Verification items for the finished model (mm, model axes). A direction names the side the tool comes from. Round coordinates to 2 decimals unless told otherwise and drop trailing zeros. Loops run counter-clockwise (first coordinate to the right, second up) from the corner with the lowest first, then second, coordinate; pieces in that order, holes last. Notation, with made-up numbers: (10, 3) -> (56, 3) arc R14 ccw to (56, 20) -> close; hole circle Ø6 at (84.5, -39). An arc over 180 degrees is marked (long way). Use a Markdown table: item, result. Add a question column.
```python
from build123d import *

# Parameters (mm, degrees)
SKETCH1_W           = 45
SKETCH1_H           = 20
BOSS_EXTRUDE1_DEPTH = 1
SKETCH2_R           = 8.5
BOSS_EXTRUDE2_DEPTH = 10
SKETCH3_R           = 7
CUT_EXTRUDE1_DEPTH  = 1
SKETCH4_W           = 1
SKETCH4_H           = 7
BOSS_EXTRUDE3_DEPTH = 1


with BuildPart() as part:
    # Sketch1 → Boss-Extrude1 (new body)
    with BuildSketch(Plane(origin=(0, 0, 0), x_dir=(1, 0, 0), z_dir=(0, 1, 0))):
        Rectangle(SKETCH1_W, SKETCH1_H)
    extrude(amount=BOSS_EXTRUDE1_DEPTH)

    # Sketch2 → Boss-Extrude2 (add)
    with BuildSketch(Plane(origin=(0, 1, 0), x_dir=(1, 0, 0), z_dir=(0, 1, 0))):
        with Locations(Location((-13, 0, 0), (0, 0, 270))):
            Circle(SKETCH2_R)
        with Locations(Location((13, 0, 0), (0, 0, 270))):
            Circle(SKETCH2_R)
    extrude(amount=BOSS_EXTRUDE2_DEPTH)

    # Sketch3 → Cut-Extrude1 (cut)
    with BuildSketch(Plane(origin=(0, 11, 0), x_dir=(1, 0, 0), z_dir=(0, 1, 0))):
        with Locations(Location((-13, 0, 0), (0, 0, 270))):
            Circle(SKETCH3_R)
        with Locations(Location((13, 0, 0), (0, 0, 270))):
            Circle(SKETCH3_R)
    extrude(amount=-CUT_EXTRUDE1_DEPTH, mode=Mode.SUBTRACT)

    # Sketch4 → Boss-Extrude3 (add)
    with BuildSketch(Plane(origin=(0, 1, 0), x_dir=(1, 0, 0), z_dir=(0, 1, 0))):
        with Locations((-1, 11.5)):
            Rectangle(SKETCH4_W, SKETCH4_H)
        with Locations((-3, 11.5)):
            Rectangle(SKETCH4_W, SKETCH4_H)
        with Locations((3, 11.5)):
            Rectangle(SKETCH4_W, SKETCH4_H)
        with Locations((1, 11.5)):
            Rectangle(SKETCH4_W, SKETCH4_H)
    extrude(amount=BOSS_EXTRUDE3_DEPTH)


solid = part.part
```
1) Access from +Z, -Z, +X, -X, +Y, -Y to the whole of each face (thin tool, end or side, straight path). Record for faces 4 (the face through (-0.5, 1.5, -11.5)), 5 (the face through (-13, 10, 0)), 6 (the face through (-3, 1.5, -8)), 7 (the face through (-1, 1, -13)).
2) Sectioned sample at B-B on z = 0. Enter the section's corners in (x, y).
3) Thickness scan on line 1 (X direction, y = 10.7, z = 0); line 2 (Y direction, x = -9.5, z = -5.75); line 3 (Y direction, x = 19.5, z = -7.75). Record the ranges inside material, lowest first.
4) Sectioned sample at C-C on y = 5. Enter the section's corners in (x, z), then the cut area to 3 significant figures.
5) Sectioned sample at A-A on x = 13. Enter the section's corners in (y, z), then the cut area to 3 significant figures.
6) Sectioned sample at D-D on x = -16.5. Enter the section's corners in (y, z), then the cut area to 3 significant figures.
7) Go/stop test with flat-tipped pins: pin 1 (5 mm diameter, centred on x = 6, y = 2.5, fed in from -Z); pin 2 (1 mm diameter, centred on y = 7.5, z = -7.5, fed in from -X); pin 3 (0.8 mm diameter, centred on x = -1, z = -10, fed in from +Y). Record where each tip stops, or that it passes through.
8) Release check for a two-part mould opening along X. For faces 1 (the face through (1.5, 1.5, -11.5)), 2 (the face through (-3, 1.5, -15)), 3 (the face through (22.5, 0.5, 0.1)) record: released by +X, released by -X, zero draft, split by the parting line, or undercut.
Geometry results:
| question | item | result |
|---|---|---|
| 1 | face 4 | +Z, -Z, +Y |
| 1 | face 5 | +Y |
| 1 | face 6 | +Z, +Y |
| 1 | face 7 | -Z, +X, -X, -Y |
| 2 | outline | (-22.5, 0) -> (22.5, 0) -> (22.5, 1) -> (21.5, 1) -> (21.5, 11) -> (20, 11) -> (20, 10) -> (6, 10) -> (6, 11) -> (4.5, 11) -> (4.5, 1) -> (-4.5, 1) -> (-4.5, 11) -> (-6, 11) -> (-6, 10) -> (-20, 10) -> (-20, 11) -> (-21.5, 11) -> (-21.5, 1) -> (-22.5, 1) -> close |
| 3 | line 1 | -21.5 to -20, -6 to -4.5, 4.5 to 6, 20 to 21.5 |
| 3 | line 2 | 0 to 10 |
| 3 | line 3 | 0 to 1 |
| 4 | outline | circle Ø17 at (-13, 0); circle Ø17 at (13, 0) |
| 4 | area | 454 mm^2 |
| 5 | outline | (0, -10) -> (1, -10) -> (1, -8.5) -> (11, -8.5) -> (11, -7) -> (10, -7) -> (10, 7) -> (11, 7) -> (11, 8.5) -> (1, 8.5) -> (1, 10) -> (0, 10) -> close |
| 5 | area | 176 mm^2 |
| 6 | outline | (0, -10) -> (1, -10) -> (1, -7.75) -> (11, -7.75) -> (11, -6.06) -> (10, -6.06) -> (10, 6.06) -> (11, 6.06) -> (11, 7.75) -> (1, 7.75) -> (1, 10) -> (0, 10) -> close |
| 6 | area | 163 mm^2 |
| 7 | pin 1 | z = -10 |
| 7 | pin 2 | x = -17.82 |
| 7 | pin 3 | y = 2 |
| 8 | face 1 | undercut |
| 8 | face 2 | zero draft |
| 8 | face 3 | released by +X |
